Geometry: final body of the model. Coordinates: model frame, mm. A direction names the side the tool comes from. Coordinates: 2 decimals unless noted, no trailing zeros. Loops run counter-clockwise (first coordinate to the right, second up) from the corner with the lowest first, then second, coordinate; pieces in that order, holes last. Notation, with made-up numbers: (17.5, 86) - (70.5, 86) arc R25 ccw to (70.5, 119) - close; hole circle Ø3 at (4.5, -12). An arc over 180 degrees is marked (long way). Return JSON: item names as keys, results as strings.
from build123d import *

# Parameters (mm, degrees)
F0_W     = 20
F0_H     = 140
F0_W_2   = 320
F1_DEPTH = 20
F2_W     = 10
F2_H     = 140
F3_DEPTH = 20
F5_DEPTH = 10


with BuildPart() as f1:
    # F0 (on Front) → F1 (new body)
    with BuildSketch(Plane.XZ):
        with Locations((-330, 70)):
            Rectangle(F0_W, F0_H)
        with Locations((-160, 70)):
            Rectangle(F0_W_2, F0_H)
    extrude(amount=F1_DEPTH)

    # F2 (on face) → F3 (cut)
    with BuildSketch(Plane.YZ):
        with Locations((-15, 70)):
            Rectangle(F2_W, F2_H)
    extrude(amount=-F3_DEPTH, mode=Mode.SUBTRACT)

    # F4 (on face) → F5 (cut)
    with BuildSketch(Plane(origin=(-340, 0, 0), x_dir=(0, -1, 0), z_dir=(-1, 0, 0))):
        with BuildLine():
            ThreePointArc((15, 37.6264154911), (10, 42.6264154911), (5, 37.6264154911))
            Line((5, 37.6264154911), (15, 37.6264154911))
        make_face()
        with BuildLine():
            Line((15, 37.6264154911), (5, 37.6264154911))
            ThreePointArc((5, 37.6264154911), (10, 32.6264154911), (15, 37.6264154911))
        make_face()
        with BuildLine():
            ThreePointArc((15, 107.6264154911), (10, 112.6264154911), (5, 107.6264154911))
            Line((5, 107.6264154911), (15, 107.6264154911))
        make_face()
        with BuildLine():
            Line((15, 107.6264154911), (5, 107.6264154911))
            ThreePointArc((5, 107.6264154911), (10, 102.6264154911), (15, 107.6264154911))
        make_face()
        with BuildLine():
            Line((15, 70), (5, 70))
            ThreePointArc((5, 70), (10, 65), (15, 70))
        make_face()
        with BuildLine():
            ThreePointArc((15, 70), (10, 75), (5, 70))
            Line((5, 70), (15, 70))
        make_face()
    extrude(amount=-F5_DEPTH, mode=Mode.SUBTRACT)


solid = f1.part
Item 1: Ray query, probe 1 along Z at (x, y) = (-337.75, -10); probe 2 along X at (y, z) = (-14.5, 91). Return the intervals inside material, ascending. Write a range as from..to.
Worked out:
{"probe 1": "0..32.63, 42.63..65, 75..102.63, 112.63..140", "probe 2": "-340..-20"}
Item 2: Section query A-A, the plane z = 70. Return loops of the section in (x, y), and give its area (3 significant figures).
Worked out:
{"outline": "(-340, -20) - (-20, -20) - (-20, -10) - (0, -10) - (0, 0) - (-340, 0) - (-340, -5) - (-330, -5) - (-330, -15) - (-340, -15) - close", "area": "6,500 mm^2"}
Item 3: Mould query, pull axis Z, two halves, no side actions, for faces 4 (the face through (-340, -3, 69)), 5 (the face through (-172, -10, 0)), 6 (the face through (-335.07, -10.65, 32.67)). Classes: +Z half, -Z half, draft (parallel to the pull), parting line (faces both ways), or undercut.
Worked out:
{"face 4": "draft", "face 5": "-Z half", "face 6": "undercut"}
Item 4: Reachability of faces 1 (the face through (-335.07, -7.31, 103.41)), 2 (the face through (-20, -15, 71)), 3 (the face through (-182, -20, 71)) from +Z, -Z, +X, -X, +Y, -Y: full face, straight path, thin tool, end or side. Return the list, or none.
Worked out:
{"face 1": "-X", "face 2": "+Z, -Z, +X, -Y", "face 3": "+Z, -Z, +X, -X, -Y"}
Item 5: First-contact query: pin 1 Ø10 at (x, z) = (-9, 100.5) entering from -Y; pin 2 Ø8 at (y, z) = (-10, 70) entering from -X; pin 3 Ø5 at (y, z) = (-13, 96.5) entering from +X. Flat tips, straight axial feed; report the tip coordinate or a pass-through.
Worked out:
{"pin 1": "y = -10", "pin 2": "x = -330", "pin 3": "x = -20"}
